```python
from build123d import *

# Parameters (mm, degrees)
CROQUIS1_R              = 1.75
SALIENTE_EXTRUIR1_DEPTH = 4


with BuildPart() as part:
    # Croquis1 → Saliente-Extruir1 (new body)
    with BuildSketch(Plane(origin=(0, 0, 0), x_dir=(1, 0, 0), z_dir=(0, 1, 0))):
        with BuildLine():
            Line((-11.167093962, 2.499461471), (11.171906038, 2.499461471))
            add(Edge.make_bspline(
                [(11.171906038, 2.499461471), (12.207826719, 2.608902185), (13.014633598, 3.14028172)],
                knots=[0, 0, 0, 0.652329484, 0.652329484, 0.652329484], degree=2))
            ThreePointArc((13.014633598, 3.14028172), (19.501897093, 0.016094387), (13.027906038, -3.135504249))
            add(Edge.make_bspline(
                [(11.171906038, -2.500538529), (12.163350933, -2.700124356), (13.027906038, -3.135504249)],
                knots=[0, 0, 0, 0.381033485, 0.381033485, 0.381033485], degree=2))
            Line((11.171906038, -2.500538529), (-11.176720188, -2.500538529))
            add(Edge.make_bspline(
                [(-11.176720188, -2.500538529), (-12.181502866, -2.673255137), (-13.0255, -3.143139195)],
                knots=[0, 0, 0, 0.480047459, 0.480047459, 0.480047459], degree=2))
            ThreePointArc((-13.0255, -3.143139195), (-19.4995, 0), (-13.0255, 3.143139195))
            add(Edge.make_bspline(
                [(-11.167093962, 2.499461471), (-12.150237992, 2.727686633), (-13.0255, 3.143139195)],
                knots=[0, 0, 0, 0.309192528, 0.309192528, 0.309192528], degree=2))
        make_face()
        with Locations((-15.4995, 0)):
            Circle(CROQUIS1_R, mode=Mode.SUBTRACT)
        with Locations((15.501906038, 0.007634946)):
            Circle(CROQUIS1_R, mode=Mode.SUBTRACT)
    extrude(amount=SALIENTE_EXTRUIR1_DEPTH)


solid = part.part
```
Can you work these out from the model? Positions are in its coordinate system, mm. A direction names the side the tool comes from. Give positions to 0.01 mm unless a question says otherwise; leave off trailing zeros. Loops run counter-clockwise (first coordinate to the right, second up) from the corner with the lowest first, then second, coordinate; pieces in that order, holes last. Notation, with made-up numbers: M 28,-23.75 L 59,-23.75 A20 cw 59,-2.75 Z; hole C 56.5,-27.75 d11. An arc over 180 degrees is marked long. Use CSV: the item, a comma, the result in double quotes. Start each with the question number.
1. If we mould it in two halves opening along X, with no side actions, what happens to faces 1 (the face through (-17.248, 1.972, -0.077)), 2 (the face through (0, 0, 0)), 3 (the face through (0, 2, 2.501))? For each: released by +X, released by -X, zero draft, split by the parting line, or undercut.
2. Imagine slicing it at C-C, the plane y = 0.85. Count the separate pieces of the cut face and the enclosed holes in it, plus the area to 3 significant figures.
3. For P1, Ø1.5, axis at x = 12, y = 1, coming from the -Z side; P2, Ø1.5, axis at y = 2.5, z = 2, coming from the +X side; P3, Ø1, axis at x = -14, y = 2.5, coming from the +Z side, each with a flat end and sliding along its axis, tell me the tip position at first contact or that it passes through.
4. Imagine slicing it at A-A, the plane z = -0.5. Write out the boundary of the cut face in (x, y), plus the area to 3 significant figures.
5. Imagine slicing it at D-D, the plane z = 1.25. Write out the boundary of the cut face in (x, y) (3 decimals).
6. Imagine slicing it at B-B, the plane x = -7. Write out the boundary of the cut face in (y, z).
7. If I drill on L1, parallel to X at y = 2.1, z = 0.75; L2, parallel to Z at x = -15.5, y = 3.15; L3, parallel to X at y = 2.95, z = -1.5, over which ranges is the centre line in solid material (lowest first)?
8. On a 3-axis mill with a long thin cutter (end or side, diameter ignored), from which of +Z, -Z, +X, -X, +Y, -Y can I reach the whole of each face in a straight line? I mean faces 4 (the face through (19.5, 2, -0.1)), 5 (the face through (0, 2, -2.499)). Say none if no direction works.
Response values:
1,face 1,"undercut"
1,face 2,"zero draft"
1,face 3,"undercut"
2,separate pieces,"1"
2,enclosed holes,"2"
2,area,"200 mm^2"
3,P1,"z = -2.98"
3,P2,"x = 19.3"
3,P3,"z = 3.87"
4,outline,"M -19.47,0 L -17.18,0 L -17.18,4 L -19.47,4 Z; M -13.82,0 L 13.82,0 L 13.82,4 L -13.82,4 Z; M 17.18,0 L 19.47,0 L 19.47,4 L 17.18,4 Z"
4,area,"129 mm^2"
5,outline,"M -19.299,0 L -16.724,0 L -16.724,4 L -19.299,4 Z; M -14.275,0 L 14.285,0 L 14.285,4 L -14.275,4 Z; M 16.719,0 L 19.299,0 L 19.299,4 L 16.719,4 Z"
6,outline,"M 0,-2.5 L 4,-2.5 L 4,2.5 L 0,2.5 Z"
7,L1,"-19.43 to -17.08, -13.92 to 13.92, 17.08 to 19.43"
7,L2,"-4 to -1.75, 1.75 to 4"
7,L3,"-19.21 to -16.4, -14.6 to 14.59, 16.42 to 19.21"
8,face 4,"+Y, -Y"
8,face 5,"-Z, +Y, -Y"
